from build123d import *

# Parameters (mm, degrees)
SKETCH1_W           = 260
SKETCH1_H           = 64
BOSS_EXTRUDE1_DEPTH = 11
CUT_EXTRUDE1_DEPTH  = 22
BOSS_EXTRUDE2_DEPTH = 65
CUT_EXTRUDE2_DEPTH  = 164.621514478
CUT_EXTRUDE3_DEPTH  = 96
SKETCH6_R           = 9.5
CUT_EXTRUDE4_DEPTH  = 96
SKETCH7_R           = 15
CUT_EXTRUDE5_DEPTH  = 12
CUT_EXTRUDE7_START  = -12
CUT_EXTRUDE7_DEPTH  = 38
CHAMFER1_SIZE       = 2
CHAMFER2_SIZE       = 2
SKETCH13_W          = 114
SKETCH13_H          = 40
CUT_EXTRUDE8_DEPTH  = 2


with BuildPart() as part:
    # Sketch1 → Boss-Extrude1 (new, symmetric)
    with BuildSketch(Plane(origin=(0, 0, 0), x_dir=(1, 0, 0), z_dir=(0, 1, 0))):
        Rectangle(SKETCH1_W, SKETCH1_H)
    extrude(amount=BOSS_EXTRUDE1_DEPTH, both=True)

    # Sketch2 → Cut-Extrude1 (cut)
    with BuildSketch(Plane(origin=(0, 11, 0), x_dir=(1, 0, 0), z_dir=(0, 1, 0))):
        with BuildLine():
            Line((-108, 8), (-102, 8))
            ThreePointArc((-102, 8), (-94, 0), (-102, -8))
            Line((-102, -8), (-108, -8))
            ThreePointArc((-108, -8), (-116, 0), (-108, 8))
        make_face()
        with BuildLine():
            Line((108, 8), (102, 8))
            ThreePointArc((102, 8), (94, 0), (102, -8))
            Line((102, -8), (108, -8))
            ThreePointArc((108, -8), (116, 0), (108, 8))
        make_face()
    extrude(amount=-CUT_EXTRUDE1_DEPTH, mode=Mode.SUBTRACT)

    # Sketch3 → Boss-Extrude2 (add)
    with BuildSketch(Plane(origin=(0, 11, 0), x_dir=(1, 0, 0), z_dir=(0, 1, 0))):
        with BuildLine():
            Line((-64.498061986, 32), (64.498061986, 32))
            ThreePointArc((64.498061986, 32), (72, 0), (64.498061986, -32))
            Line((64.498061986, -32), (-64.498061986, -32))
            ThreePointArc((-64.498061986, -32), (-72, 0), (-64.498061986, 32))
        make_face()
    extrude(amount=BOSS_EXTRUDE2_DEPTH)

    # Sketch4 → Cut-Extrude2 (cut, through all)
    with BuildSketch(Plane.XY.offset(32)):
        Polygon((-130, 11), (-128, 11), (-130, -11), align=None)
        Polygon((130, -11), (128, 11), (130, 11), align=None)
    extrude(amount=-CUT_EXTRUDE2_DEPTH, mode=Mode.SUBTRACT)

    # Sketch5 → Cut-Extrude3 (cut)
    with BuildSketch(Plane.XY.offset(32)):
        with BuildLine():
            Line((-19.974984355, 76), (-36, 76))
            Line((-36, 76), (-36, 51))
            Line((-36, 51), (-32, 51))
            ThreePointArc((-32, 51), (0, 19), (32, 51))
            Line((32, 51), (36, 51))
            Line((36, 51), (36, 76))
            Line((36, 76), (-19.974984355, 76))
        make_face()
    extrude(amount=-CUT_EXTRUDE3_DEPTH, mode=Mode.SUBTRACT)

    # Sketch6 → Cut-Extrude4 (cut)
    with BuildSketch(Plane(origin=(0, 76, 0), x_dir=(1, 0, 0), z_dir=(0, 1, 0))):
        with Locations(Location((-52.5, 0, 0), (0, 0, 270))):
            Circle(SKETCH6_R)
        with Locations(Location((52.5, 0, 0), (0, 0, 90))):
            Circle(SKETCH6_R)
    extrude(amount=-CUT_EXTRUDE4_DEPTH, mode=Mode.SUBTRACT)

    # Sketch7 → Cut-Extrude5 (cut)
    with BuildSketch(Plane.XZ.offset(11)):
        with Locations(Location((-52.5, 0, 0), (0, 0, 270))):
            Circle(SKETCH7_R)
        with Locations(Location((52.5, 0, 0), (0, 0, 270))):
            Circle(SKETCH7_R)
    extrude(amount=-CUT_EXTRUDE5_DEPTH, mode=Mode.SUBTRACT)

    # Sketch10 → Cut-Extrude7 (cut)
    with BuildSketch(Plane.XY.offset(32).offset(CUT_EXTRUDE7_START)):
        with BuildLine():
            Line((-34, 51), (34, 51))
            ThreePointArc((34, 51), (0, 17), (-34, 51))
        make_face()
    extrude(amount=-CUT_EXTRUDE7_DEPTH, mode=Mode.SUBTRACT)

    # Chamfer1
    chamfer1_edges = [part.edges().sort_by_distance(p)[0] for p in [
        (0, 19, 20),
    ]]
    chamfer(chamfer1_edges, length=CHAMFER1_SIZE - 0.0001)  # a hair under: the kernel refuses the full size

    # Chamfer2
    chamfer2_edges = [part.edges().sort_by_distance(p)[0] for p in [
        (0, 19, -18),
    ]]
    chamfer(chamfer2_edges, length=CHAMFER2_SIZE - 0.0001)  # a hair under: the kernel refuses the full size

    # Sketch13 → Cut-Extrude8 (cut)
    with BuildSketch(Plane.XZ.offset(11)):
        with Locations((-61, -2.5e-06)):
            Rectangle(SKETCH13_W, SKETCH13_H)
        with Locations((61, -2.5e-06)):
            Rectangle(SKETCH13_W, SKETCH13_H)
    extrude(amount=-CUT_EXTRUDE8_DEPTH, mode=Mode.SUBTRACT)


solid = part.part
Verification items for the finished model (mm, model axes). A direction names the side the tool comes from. Round coordinates to 2 decimals unless told otherwise and drop trailing zeros. Loops run counter-clockwise (first coordinate to the right, second up) from the corner with the lowest first, then second, coordinate; pieces in that order, holes last. Notation, with made-up numbers: (9, 51.25) - (55, 51.25) arc R24 cw to (55, 68.25) - close; hole circle Ø8 at (86, -3.5). An arc over 180 degrees is marked (long way). Use a Markdown table: item, result. Add a question column.
1. Thickness scan on probe 1 along X at (y, z) = (58, 0); probe 2 along X at (y, z) = (66.5, -2); probe 3 along Z at (x, y) = (52.5, 25). Record the ranges inside material, lowest first. Write a range as [from, to].
2. Section check C-C, the plane z = 0. Give the number of separate pieces and of enclosed holes in the cut face, plus the area to 3 significant figures.
3. Section check A-A, the plane x = -52.5. Record the boundary of the cut face in (y, z).
4. Release check for a two-part mould opening along Z. For faces 6 (the face through (-105, 1, 8)), 7 (the face through (-72, 43, 0)), 8 (the face through (-2, 14, 32)), 9 (the face through (36, 63, 0)) record: released by +Z, released by -Z, zero draft, split by the parting line, or undercut.
5. Gauge pin test, flat ends, axial feed: pin 1 (2 mm diameter, centred on x = -33.5, z = 4.5, fed in from +Y); pin 2 (3 mm diameter, centred on x = -87.5, z = 0, fed in from +Y); pin 3 (17 mm diameter, centred on x = -52.5, z = 0, fed in from -Y); pin 4 (1 mm diameter, centred on y = 55.5, z = -0.5, fed in from +X). Record the tip position at first contact, or that the pin passes through.
6. Access from +Z, -Z, +X, -X, +Y, -Y to the whole of each face (thin tool, end or side, straight path). Record for faces 1 (the face through (-36, 64, 0)), 2 (the face through (-0.71, 18.69, -19.68)), 3 (the face through (-2, 14, -32)), 4 (the face through (-52, 1, -10)), 5 (the face through (-105, 1, -8)).
7. Section check B-B, the plane x = 80. Record the boundary of the cut face in (y, z).
Checks:
| question | item | result |
|---|---|---|
| 1 | probe 1 | x = [-72, -62], [-43, -36], [36, 43], [62, 72] |
| 1 | probe 2 | x = [-71.97, -61.79], [-43.21, -36], [36, 43.21], [61.79, 71.97] |
| 1 | probe 3 | z = [-32, -9.5], [9.5, 32] |
| 2 | separate pieces | 5 |
| 2 | enclosed holes | 0 |
| 2 | area | 6,630 mm^2 |
| 3 | outline | (-11, -32) - (76, -32) - (76, -9.5) - (1, -9.5) - (1, -15) - (-9, -15) - (-9, -20) - (-11, -20) - close; (-11, 20) - (-9, 20) - (-9, 15) - (1, 15) - (1, 9.5) - (76, 9.5) - (76, 32) - (-11, 32) - close |
| 4 | face 6 | undercut |
| 4 | face 7 | split by the parting line |
| 4 | face 8 | released by +Z |
| 4 | face 9 | zero draft |
| 5 | pin 1 | stops at y = 51 |
| 5 | pin 2 | stops at y = 11 |
| 5 | pin 3 | passes through |
| 5 | pin 4 | stops at x = 72 |
| 6 | face 1 | +Z, -Z, +Y |
| 6 | face 2 | +Y |
| 6 | face 3 | -Z, +X, -X, +Y, -Y |
| 6 | face 4 | -Y |
| 6 | face 5 | +Y, -Y |
| 7 | outline | (-11, -32) - (11, -32) - (11, 32) - (-11, 32) - (-11, 20) - (-9, 20) - (-9, -20) - (-11, -20) - close |
